Read the model definition and answer for the solid it produces. Units are mm, in the model's axes. A direction names the side the tool comes from. Round coordinates to 2 decimals unless told otherwise and drop trailing zeros.
from build123d import *

# Parameters (mm, degrees)
PAD_DEPTH       = 5
POCKET_DEPTH    = 5.001
SKETCH137_R     = 3
PAD001_DEPTH    = 5
SKETCH_R        = 2.5
POCKET001_DEPTH = 5.001


with BuildPart() as body:
    # Sketch135 → Pad (new body)
    with BuildSketch(Plane.XY):
        with BuildLine():
            add(Edge.make_bspline(
                [(-73.5, 101.839707), (-74.771, 49.44), (-49.529, 37.339707), (-22.686, 26.780106), (0, 26.839707)],
                knots=[0, 0, 0, 0, 0, 1, 1, 1, 1, 1], degree=4))
            Line((0, 26.839707), (0, 0))
            add(Edge.make_bspline(
                [(0, 0), (-24.669, -0.204), (-39, 6.04)],
                knots=[0, 0, 0, 1, 1, 1], degree=2))
            add(Edge.make_bspline(
                [(-39, 6.04), (-72.6, 18.986), (-79.11, 71.198)],
                knots=[0, 0, 0, 1, 1, 1], degree=2))
            add(Edge.make_bspline(
                [(-79.11, 71.198), (-80.407, 98.996)],
                knots=[0, 0, 1, 1], degree=1))
            Line((-80.407, 98.996), (-80.407, 99.34))
            ThreePointArc((-80.407, 99.34), (-81.657, 100.59), (-82.907, 99.34))
            Line((-82.907, 99.34), (-82.907, 95.34))
            ThreePointArc((-82.907, 95.34), (-86.907, 91.34), (-90.907, 95.34))
            Line((-90.907, 95.34), (-90.907, 110.839707))
            ThreePointArc((-90.907, 110.839707), (-82.2035, 119.543207), (-73.5, 110.839707))
            Line((-73.5, 110.839707), (-73.5, 101.839707))
        make_face()
    extrude(amount=PAD_DEPTH)

    # Sketch136 (on Face14 of Pad) → Pocket (cut, through all)
    with BuildSketch(Plane.XY.offset(5)):
        with BuildLine():
            ThreePointArc((-85.2035, 112.089707), (-86.4535, 110.839707), (-85.2035, 109.589707))
            Line((-85.2035, 109.589707), (-79.2035, 109.589707))
            ThreePointArc((-79.2035, 109.589707), (-77.9535, 110.839707), (-79.2035, 112.089707))
            Line((-85.2035, 112.089707), (-79.2035, 112.089707))
        make_face()
    extrude(amount=-POCKET_DEPTH, mode=Mode.SUBTRACT)

    # Sketch137 (on Face5 of Pocket) → Pad001 (join)
    with BuildSketch(Plane.XY.offset(5)):
        with Locations((-39.549752, 4.644374)):
            Circle(SKETCH137_R)
        with Locations((-80.589428, 70.950429)):
            Circle(SKETCH137_R)
        with Locations((-69.533947, 32.279444)):
            Circle(SKETCH137_R)
    extrude(amount=-PAD001_DEPTH)

    # Sketch (on Face23 of Pad001) → Pocket001 (cut, through all)
    with BuildSketch(Plane.XY.offset(5)):
        with Locations((-27, 16.839707)):
            Circle(SKETCH_R)
        with Locations((-54, 31.839707)):
            Circle(SKETCH_R)
    extrude(amount=-POCKET001_DEPTH, mode=Mode.SUBTRACT)


with BuildPart() as fusion:
    # Part__Mirroring: instance of Body
    add(body.part.mirror(Plane(origin=(0, 0, 0), x_dir=(0, -1, 0), z_dir=(1, 0, 0))))

    # Fusion: union Body
    add(body.part)


solid = fusion.part
Q1. Straight lines are drawn through the part: probe 1 along X at (y, z) = (98.5, 1.85); probe 2 along X at (y, z) = (34, 2.4); probe 3 along Y at (x, z) = (54, 2). For each, find the intervals that lie inside material, in ascending order.
Verdict:
probe 1: x = -90.91 to -82.91, -80.38 to -73.54, 73.54 to 80.38, 82.91 to 90.91
probe 2: x = -71.99 to -55.26, -52.74 to -34.22, 34.22 to 52.74, 55.26 to 71.99
probe 3: y = 14.88 to 29.34, 34.34 to 46.14
Q2. Determine the mould class of faces 4 (the flat face through (-90.907, 103, 2)), 5 (the flat face through (90.907, 103, 2)), 6 (the flat face through (82, 112.09, 3)) for opening direction X: pulls with the +X half, pulls with the -X half, needs draft (parallel to the pull), parting line crosses it, or undercut.
Verdict:
face 4: pulls with the -X half
face 5: pulls with the +X half
face 6: undercut
Q3. Which of the six approach directions +Z, -Z, +X, -X, +Y, -Y give full straight-line access (tool end or side, diameter ignored) to faces 1 (the flat face through (73.5, 106, 2)), 2 (the flat face through (6, 24, 5)), 3 (the cylindrical face through (-86.82, 91.34, 2.46))?
Verdict:
face 1: +Z, -Z, +Y
face 2: +Z, +X, -X, +Y, -Y
face 3: +Z, -Z
Q4. Flat-ended cylindrical pins translate along their axes: pin 1 Ø4 at (x, y) = (54, 31.84) entering from -Z; pin 2 Ø1.5 at (x, z) = (-82, 3) entering from -Y; pin 3 Ø1.5 at (x, z) = (41, 1.5) entering from +Y. Find the tip coordinate at first contact, or state that the pin passes through.
Verdict:
pin 1: passes through
pin 2: stops at y = 68.02
pin 3: stops at y = 37.59
Q5. Section A-A (z = 4.2) is taken. State how many separate pieces and enclosed holes the cut face has, then the cut area to 3 significant figures.
Verdict:
separate pieces: 1
enclosed holes: 6
area: 5,720 mm2
